from build123d import *
from build123d.topology import SkipClean

# Parameters (mm, degrees)
SKETCH1_R           = 16.9
BOSS_EXTRUDE1_DEPTH = 9
SKETCH3_R           = 22.5
SKETCH3_R_2         = 16.9
BOSS_EXTRUDE2_DEPTH = 19
SKETCH4_R           = 4.5
BOSS_EXTRUDE3_DEPTH = 30
CUT_EXTRUDE2_DEPTH  = 4
CUT_EXTRUDE3_DEPTH  = 138.13719408
FILLET1_R           = 10
FILLET2_R           = 10
SKETCH7_R           = 4.523289267
SKETCH7_R_2         = 4.5
CUT_EXTRUDE4_DEPTH  = 230.372382819


with BuildPart() as part:
    # Sketch1 → Boss-Extrude1 (new, symmetric)
    with BuildSketch(Plane.XY):
        with BuildLine():
            Line((-10.60459099, 68.908072309), (-16.957576671, -52.314115855))
            ThreePointArc((-16.957576671, -52.314115855), (-19.883826234, -65.373191797), (-26.953938029, -76.736110444))
            ThreePointArc((-26.953938029, -76.736110444), (-33.66260365, -87.839548775), (-36, -100.6))
            Line((-36, -100.6), (-28, -100.6))
            ThreePointArc((-28, -100.6), (0, -72.6), (28, -100.6))
            Line((28, -100.6), (36, -100.6))
            ThreePointArc((36, -100.6), (33.66260365, -87.839548775), (26.953938029, -76.736110444))
            ThreePointArc((26.953938029, -76.736110444), (19.883826234, -65.373191797), (16.957576671, -52.314115855))
            Line((16.957576671, -52.314115855), (10.60459099, 68.908072309))
            ThreePointArc((10.60459099, 68.908072309), (11.910272087, 77.724804636), (16.536877761, 85.342815662))
            ThreePointArc((16.536877761, 85.342815662), (0, 123.1), (-16.536877761, 85.342815662))
            ThreePointArc((-16.536877761, 85.342815662), (-11.910272087, 77.724804636), (-10.60459099, 68.908072309))
        make_face()
        with Locations((0, 100.6)):
            Circle(SKETCH1_R, mode=Mode.SUBTRACT)
    extrude(amount=BOSS_EXTRUDE1_DEPTH, both=True)

    # Sketch3 → Boss-Extrude2 (add, symmetric)
    # profile 1 of 2: a face of its own
    with SkipClean():  # the faces are left unmerged after this step: merging them gives an invalid solid
        with BuildSketch(Plane.XY):
            with Locations((0, 100.6)):
                Circle(SKETCH3_R)
            with Locations((0, 100.6)):
                Circle(SKETCH3_R_2, mode=Mode.SUBTRACT)
        # profile 2 of 2: a face of its own
        with BuildSketch(Plane.XY):
            with BuildLine():
                Line((-28, -100.6), (-36, -100.6))
                ThreePointArc((-36, -100.6), (0, -64.6), (36, -100.6))
                Line((36, -100.6), (28, -100.6))
                ThreePointArc((28, -100.6), (0, -72.6), (-28, -100.6))
            make_face()
        extrude(amount=BOSS_EXTRUDE2_DEPTH, both=True)

    # Sketch4 → Boss-Extrude3 (add)
    with SkipClean():  # the faces are left unmerged after this step: merging them gives an invalid solid
        with BuildSketch(Plane.XZ.offset(100.6)):
            with BuildLine():
                Line((-28, 8.968695557), (28, 8.968695557))
                Line((28, 8.968695557), (38.75, 8.968695557))
                ThreePointArc((38.75, 8.968695557), (47, 0), (38.75, -8.968695557))
                Line((38.75, -8.968695557), (28, -8.968695557))
                Line((28, -8.968695557), (-28, -8.968695557))
                Line((-28, -8.968695557), (-38.75, -8.968695557))
                ThreePointArc((-38.75, -8.968695557), (-47, 0), (-38.75, 8.968695557))
                Line((-38.75, 8.968695557), (-28, 8.968695557))
            make_face()
            with Locations(Location((38, 0, 0), (0, 0, 270))):
                Circle(SKETCH4_R, mode=Mode.SUBTRACT)
            with Locations(Location((-38, 0, 0), (0, 0, 270))):
                Circle(SKETCH4_R, mode=Mode.SUBTRACT)
        extrude(amount=-BOSS_EXTRUDE3_DEPTH)

    # Sketch5 → Cut-Extrude2 (cut)
    with SkipClean():  # the faces are left unmerged after this step: merging them gives an invalid solid
        with BuildSketch(Plane.XY.offset(9)):
            with BuildLine():
                Line((-8, 45), (-8, -45))
                ThreePointArc((-8, -45), (0, -53), (8, -45))
                Line((8, -45), (8, 45))
                ThreePointArc((8, 45), (0, 53), (-8, 45))
            make_face()
        cut_extrude2 = extrude(amount=-CUT_EXTRUDE2_DEPTH, mode=Mode.SUBTRACT)

    # Mirror1: Cut-Extrude2 across plane
    with SkipClean():  # the faces are left unmerged after this step: merging them gives an invalid solid
        add(cut_extrude2.mirror(Plane.XY), mode=Mode.SUBTRACT)

    # Sketch6 → Cut-Extrude3 (cut, through all)
    with SkipClean():  # the faces are left unmerged after this step: merging them gives an invalid solid
        with BuildSketch(Plane.XY.offset(19)):
            with BuildLine():
                Line((28, -100.6), (-28, -100.6))
                ThreePointArc((-28, -100.6), (0, -72.6), (28, -100.6))
            make_face()
        extrude(amount=-CUT_EXTRUDE3_DEPTH, mode=Mode.SUBTRACT)

    # Fillet1
    fillet1_edges = [part.edges().sort_by_distance(p)[0] for p in [
        (22.483530605, -70.6, 0),
    ]]
    fillet(fillet1_edges, radius=FILLET1_R)

    # Fillet2
    fillet2_edges = [part.edges().sort_by_distance(p)[0] for p in [
        (-22.483530605, -70.6, 0),
    ]]
    fillet(fillet2_edges, radius=FILLET2_R)

    # Sketch7 → Cut-Extrude4 (cut, through all)
    with SkipClean():  # the faces are left unmerged after this step: merging them gives an invalid solid
        with BuildSketch(Plane.XZ.offset(100.6)):
            with Locations((-38, 0)):
                Circle(SKETCH7_R)
            with Locations(Location((38, 0, 0), (0, 0, 270))):
                Circle(SKETCH7_R_2)
        extrude(amount=-CUT_EXTRUDE4_DEPTH, mode=Mode.SUBTRACT)
    add(part.part.scale(1), mode=Mode.REPLACE)  # the faces are merged on a copy


solid = part.part
Could you check a few things on this model? Use its own coordinates, in mm. A direction names the side the tool comes from. Give positions to 0.01 mm unless a question says otherwise; leave off trailing zeros. Order: outer loops, then holes, each group sorted by start corner. A loop starts at its lowest first (then second) coordinate and runs counter-clockwise, first axis right, second up.
1. We'd pull the mould along Y, two halves only. Please class faces 1 (the flat face through (33, -100.6, 0)), 2 (the cylindrical face through (0, -53, -7)), 3 (the cylindrical face through (-47, -86, 0)): pulls with the +Y half, pulls with the -Y half, needs draft (parallel to the pull), parting line crosses it, or undercut.
2. I need wall thicknesses on L1, parallel to Y at x = 0, z = 13.5; L2, parallel to Y at x = -4, z = 14; L3, parallel to Z at x = 5.5, y = -14. Which ranges of each line are inside material? Lowest first, please.
3. For faces 4 (the flat face through (-8, 1, -7)), 5 (the flat face through (-2, -72, -19)), 6 (the cylindrical face through (0, 53, 7)), 7 (the cylindrical face through (-22.967, -68.755, 0.126)), which set-ups out of +Z, -Z, +X, -X, +Y, -Y let a thin tool reach every point of the face, with its end or its side?
4. Will these pins go through, and if not, where does the flat tip stop? P1, Ø13, axis at x = -1, y = -9, coming from the -Z side; P2, Ø3, axis at y = 12, z = 8.5, coming from the -X side; P3, Ø2, axis at x = 3, z = 0.5, coming from the -Y side; P4, Ø1.5, axis at x = 34, z = -0.5, coming from the -Y side.
5. Suppose I cut it at B-B (x = 13). List the corners of the cut face in (y, z) for me, plus the area to 3 significant figures.
6. Suppose I cut it at C-C (y = 35). List the corners of the cut face in (x, z) for me, plus the area to 3 significant figures.
7. Suppose I cut it at A-A (z = -13.5). List the corners of the cut face in (x, y) for me, plus the area to 3 significant figures.
8. Suppose I cut it at D-D (x = 2). List the corners of the cut face in (y, z) for me.
Solved:
1. face 1: pulls with the -Y half
1. face 2: undercut
1. face 3: needs draft
2. L1: y = -72.6 to -64.6, 78.1 to 83.7, 117.5 to 123.1
2. L2: y = -72.89 to -64.82, 78.46 to 84.18, 117.02 to 122.74
2. L3: z = -5 to 5
3. face 4: -Z
3. face 5: -Z, +X, -X, +Y, -Y
3. face 6: +Z
3. face 7: +Z, -Z, -X
4. P1: stops at z = -5
4. P2: stops at x = -13.67
4. P3: stops at y = -72.89
4. P4: stops at y = -100.6
5. outline: (-75.8, -19) - (-67.03, -19) - (-67.03, -9) - (23.2, -9) - (23.2, 9) - (-67.03, 9) - (-67.03, 19) - (-75.8, 19) - close; (80.25, -9) - (82.24, -9) - (82.24, -19) - (89.8, -19) - (89.8, 19) - (82.24, 19) - (82.24, 9) - (80.25, 9) - close; (111.4, -19) - (118.96, -19) - (118.96, 19) - (111.4, 19) - close
5. area: 2,570 mm2
6. outline: (-12.38, -9) - (-8, -9) - (-8, -5) - (8, -5) - (8, -9) - (12.38, -9) - (12.38, 9) - (8, 9) - (8, 5) - (-8, 5) - (-8, 9) - (-12.38, 9) - close
6. area: 318 mm2
7. outline: (-36, -100.6) - (-28, -100.6) arc R28 cw to (28, -100.6) - (36, -100.6) arc R36 ccw to start; circle Ø45 at (0, 100.6); hole circle Ø33.8 at (0, 100.6)
7. area: 1,500 mm2
8. outline: (-72.67, -19) - (-64.66, -19) - (-64.66, -9) - (-52.75, -9) - (-52.75, -5) - (52.75, -5) - (52.75, -9) - (78.19, -9) - (78.19, -19) - (83.82, -19) - (83.82, 19) - (78.19, 19) - (78.19, 9) - (52.75, 9) - (52.75, 5) - (-52.75, 5) - (-52.75, 9) - (-64.66, 9) - (-64.66, 19) - (-72.67, 19) - close; (117.38, -19) - (123.01, -19) - (123.01, 19) - (117.38, 19) - close
